from build123d import *

# Parameters (mm, degrees)
F0_W     = 3.85
F0_H     = 3.202905
F1_DEPTH = 25


with BuildPart() as f1:
    # F0 (on Top) → F1 (new body)
    with BuildSketch(Plane.XY):
        with BuildLine():
            Line((0, 11.35), (0, 13.15))
            Line((0, 13.15), (-3.85, 13.15))
            Line((-3.85, 13.15), (-10.455501, 13.15))
            ThreePointArc((-10.455501, 13.15), (-16.789703, 0.588121), (-11.35, -12.386182))
            Line((-11.35, -12.386182), (-11.35, 0))
            ThreePointArc((-11.35, 0), (-8.025662, 8.025662), (0, 11.35))
        make_face()
        with BuildLine():
            ThreePointArc((11.35, -12.386182), (15.377256, -6.766092), (16.8, 0))
            ThreePointArc((16.8, 0), (15.130969, 7.30026), (10.455501, 13.15))
            Line((10.455501, 13.15), (3.85, 13.15))
            Line((3.85, 13.15), (0, 13.15))
            Line((0, 13.15), (0, 11.35))
            ThreePointArc((0, 11.35), (8.025662, 8.025662), (11.35, 0))
            Line((11.35, 0), (11.35, -12.386182))
        make_face()
        with Locations((-1.925, 14.751452)):
            Rectangle(F0_W, F0_H)
        with Locations((1.925, 14.751452)):
            Rectangle(F0_W, F0_H)
    extrude(amount=F1_DEPTH)


solid = f1.part
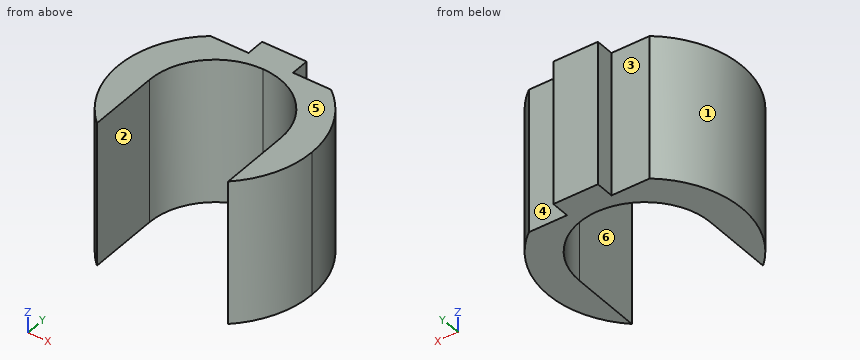
Could you check a few things on this model? Use its own coordinates, in mm. Face numbers are marked on the shaded views. A direction names the side the tool comes from. Give positions to 0.01 mm unless a question says otherwise; leave off trailing zeros. Order: outer loops, then holes, each group sorted by start corner. A loop starts at its lowest first (then second) coordinate and runs counter-clockwise, first axis right, second up. Notation, with made-up numbers: (27.5, 87) -> (80.5, 87) arc R11 cw to (80.5, 104) -> close; hole circle Ø5 at (70.25, 28.5). An arc over 180 degrees is marked (long way). Return JSON: item names as keys, results as strings.
1. On a 3-axis mill with a long thin cutter (end or side, diameter ignored), from which of +Z, -Z, +X, -X, +Y, -Y can I reach the whole of each face in a straight line? I mean the marked faces 4, 5 and 6. Say none if no direction works.
Answer list:
{"face 4": "+Z, -Z, +X, +Y", "face 5": "+Z, +X, -X, +Y, -Y", "face 6": "+Z, -Z, -Y"}
2. Imagine slicing it at C-C on y = 6.5. List the corners of the cut face in (x, z) for me, then the cut area to 3 significant figures.
Answer list:
{"outline": "(-15.49, 0) -> (-9.3, 0) -> (-9.3, 25) -> (-15.49, 25) -> close; (9.3, 0) -> (15.49, 0) -> (15.49, 25) -> (9.3, 25) -> close", "area": "309 mm2"}
3. For pin 1 Ø4 at (x, z) = (-6, 5) entering from +Y; pin 2 Ø3.5 at (y, z) = (15, 12.5) entering from -X; pin 3 Ø6 at (y, z) = (-9, 18.5) entering from -X; pin 4 Ø6 at (x, y) = (7.5, 11) entering from -Z, each with a flat end and sliding along its axis, tell me the tip position at first contact or that it passes through.
Answer list:
{"pin 1": "stops at y = 13.15", "pin 2": "stops at x = -3.85", "pin 3": "stops at x = -15.69", "pin 4": "stops at z = 0"}
4. I need wall thicknesses on line 1 (X direction, y = 4.75, z = 7.25); line 2 (X direction, y = 1, z = 21); line 3 (Y direction, x = 0, z = 6.5). Which ranges of each line are inside material? Lowest first, please. Write a range as from..to.
Answer list:
{"line 1": "x = -16.11..-10.31, 10.31..16.11", "line 2": "x = -16.77..-11.31, 11.31..16.77", "line 3": "y = 11.35..16.35"}
5. Thinking about a two-plate mould opening in X: for the marked faces 1, 2 and 3, which applies, pulls with the +X half, pulls with the -X half, needs draft (parallel to the pull), parting line crosses it, or undercut?
Answer list:
{"face 1": "pulls with the -X half", "face 2": "undercut", "face 3": "needs draft"}
6. Imagine slicing it at D-D on x = -6. List the corners of the cut face in (y, z) for me, then the cut area to 3 significant figures.
Answer list:
{"outline": "(9.63, 0) -> (13.15, 0) -> (13.15, 25) -> (9.63, 25) -> close", "area": "87.9 mm2"}
7. Imagine slicing it at B-B on z = 8.5. List the corners of the cut face in (x, y) for me, then the cut area to 3 significant figures.
Answer list:
{"outline": "(-11.35, -12.39) -> (-11.35, 0) arc R11.35 cw to (11.35, 0) -> (11.35, -12.39) arc R16.8 ccw to (16.8, 0) arc R16.8 ccw to (10.46, 13.15) -> (3.85, 13.15) -> (3.85, 16.35) -> (-3.85, 16.35) -> (-3.85, 13.15) -> (-10.46, 13.15) arc R16.8 ccw to start", "area": "307 mm2"}
8. Imagine slicing it at A-A on y = -4.5. List the corners of the cut face in (x, z) for me.
Answer list:
{"outline": "(-16.19, 0) -> (-11.35, 0) -> (-11.35, 25) -> (-16.19, 25) -> close; (11.35, 0) -> (16.19, 0) -> (16.19, 25) -> (11.35, 25) -> close"}
